Geometry: final body of the model. Coordinates: model frame, mm. A direction names the side the tool comes from. Coordinates: 2 decimals unless noted, no trailing zeros. Loops run counter-clockwise (first coordinate to the right, second up) from the corner with the lowest first, then second, coordinate; pieces in that order, holes last. Notation, with made-up numbers: (43, 58.25) - (82, 58.25) arc R18 ccw to (82, 83.25) - close; hole circle Ø6 at (38.25, 49.5). An arc over 180 degrees is marked (long way). Put each result on its own line as item: value. Start each with the question number.
1) Draft query along Y for faces 1 (the flat face through (50, 5, 0)), 2 (the cylindrical face through (0, 50, 0)), 3 (the flat face through (45, 0, 0)), 4 (the cylindrical face through (-2.17, 20.24, -0.28)). Return one class per face: +Y half, -Y half, draft (parallel to the pull), parting line (faces both ways), or undercut.
2) Section A-A on x = 0. Output: boundary loops of the cut face in (y, z).
3) Section B-B on z = -14. Output: boundary loops of the cut face in (x, y), and give its area (3 significant figures).
4) Material intervals for line 1 along Y through (x, z) = (0, -6.5); line 2 along X through (y, z) = (30.5, 16); line 3 along X through (y, z) = (17.5, 3), sorted ascending. Write a range as from..to.
5) Contact query for flat-ended pins moving along their axis: pin 1 Ø2 at (x, z) = (22.5, -8) entering from +Y; pin 2 Ø6 at (y, z) = (33.5, -15.5) entering from -X; pin 3 Ø4 at (y, z) = (32.5, 16) entering from +X. Output: stop coordinate, or through.
6) Section D-D on x = -30. Output: boundary loops of the cut face in (y, z).
7) Section C-C on y = 15. Output: boundary loops of the cut face in (x, z).
8) Reachability of faces 5 (the flat face through (-20, 20, 0)), 6 (the flat face through (-1, 5, 0)), 7 (the flat face through (20, 20, 0)) from +Z, -Z, +X, -X, +Y, -Y: full face, straight path, thin tool, end or side. Return the list, or none.
```python
from build123d import *

# Parameters (mm, degrees)
SKETCH1_R           = 10
BOSS_EXTRUDE1_DEPTH = 20


with BuildPart() as part:
    # Sketch1 → Boss-Extrude1 (new, symmetric)
    with BuildSketch(Plane.XY):
        with BuildLine():
            Line((50, 0), (50, 10))
            Line((50, 10), (20, 10))
            Line((20, 10), (20, 30))
            ThreePointArc((20, 30), (0, 50), (-20, 30))
            Line((-20, 30), (-20, 10))
            Line((-20, 10), (-50, 10))
            Line((-50, 10), (-50, 0))
            Line((-50, 0), (-40, 0))
            Line((-40, 0), (-40, 5))
            Line((-40, 5), (40, 5))
            Line((40, 5), (40, 0))
            Line((40, 0), (50, 0))
        make_face()
        with Locations((0, 30)):
            Circle(SKETCH1_R, mode=Mode.SUBTRACT)
    extrude(amount=BOSS_EXTRUDE1_DEPTH, both=True)


solid = part.part
```
Answer block:
1. face 1: draft
1. face 2: +Y half
1. face 3: -Y half
1. face 4: undercut
2. outline: (5, -20) - (20, -20) - (20, 20) - (5, 20) - close; (40, -20) - (50, -20) - (50, 20) - (40, 20) - close
3. outline: (-50, 0) - (-40, 0) - (-40, 5) - (40, 5) - (40, 0) - (50, 0) - (50, 10) - (20, 10) - (20, 30) arc R20 ccw to (-20, 30) - (-20, 10) - (-50, 10) - close; hole circle Ø20 at (0, 30)
3. area: 1,710 mm²
4. line 1: y = 5..20, 40..50
4. line 2: x = -19.99..-9.99, 9.99..19.99
4. line 3: x = -20..20
5. pin 1: stops at y = 10
5. pin 2: stops at x = -19.99
5. pin 3: stops at x = 19.99
6. outline: (5, -20) - (10, -20) - (10, 20) - (5, 20) - close
7. outline: (-20, -20) - (20, -20) - (20, 20) - (-20, 20) - close
8. face 5: +Z, -Z, -X, +Y
8. face 6: +Z, -Z, -Y
8. face 7: +Z, -Z, +X, +Y
